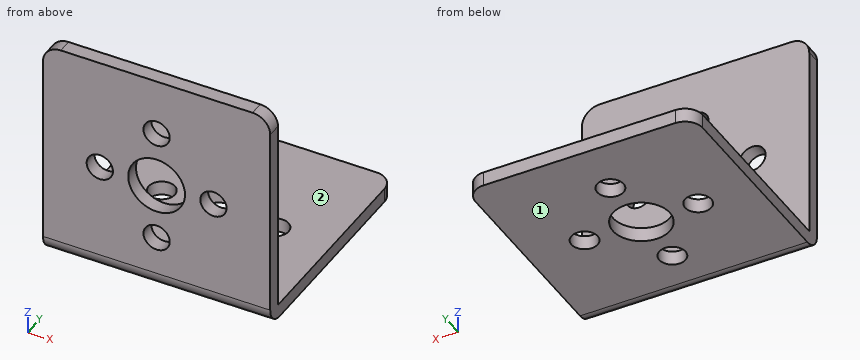
from build123d import *

# Parameters (mm, degrees)
SKETCH1_W           = 32
SKETCH1_H           = 32
BOSS_EXTRUDE1_DEPTH = 16
SKETCH2_W           = 30
SKETCH2_H           = 30
CUT_EXTRUDE1_DEPTH  = 32
SKETCH3_R           = 4
SKETCH3_R_2         = 1.85
CUT_EXTRUDE2_DEPTH  = 33
SKETCH4_R           = 4
SKETCH4_R_2         = 1.85
CUT_EXTRUDE3_DEPTH  = 33
FILLET1_R           = 2.5


with BuildPart() as part:
    # Sketch1 → Boss-Extrude1 (new body, symmetric)
    with BuildSketch(Plane(origin=(0, 0, 0), x_dir=(0, 0, -1), z_dir=(1, 0, 0))):
        Rectangle(SKETCH1_W, SKETCH1_H)
    extrude(amount=BOSS_EXTRUDE1_DEPTH, both=True)

    # Sketch2 → Cut-Extrude1 (cut)
    with BuildSketch(Plane(origin=(16, 0, 0), x_dir=(0, 0, -1), z_dir=(1, 0, 0))):
        with Locations((-1, 1)):
            Rectangle(SKETCH2_W, SKETCH2_H)
    extrude(amount=-CUT_EXTRUDE1_DEPTH, mode=Mode.SUBTRACT)

    # Sketch3 → Cut-Extrude2 (cut, through all)
    with BuildSketch(Plane(origin=(0, 0, -16), x_dir=(-1, 0, 0), z_dir=(0, 0, -1))):
        Circle(SKETCH3_R)
        with Locations((8, 0)):
            Circle(SKETCH3_R_2)
        with Locations((-8, 0)):
            Circle(SKETCH3_R_2)
        with Locations((0, 8)):
            Circle(SKETCH3_R_2)
        with Locations((0, -8)):
            Circle(SKETCH3_R_2)
    extrude(amount=-CUT_EXTRUDE2_DEPTH, mode=Mode.SUBTRACT)

    # Sketch4 → Cut-Extrude3 (cut, through all)
    with BuildSketch(Plane.XZ.offset(16)):
        Circle(SKETCH4_R)
        with Locations((8, 0)):
            Circle(SKETCH4_R_2)
        with Locations((-8, 0)):
            Circle(SKETCH4_R_2)
        with Locations((0, 8)):
            Circle(SKETCH4_R_2)
        with Locations((0, -8)):
            Circle(SKETCH4_R_2)
    extrude(amount=-CUT_EXTRUDE3_DEPTH, mode=Mode.SUBTRACT)

    # Fillet1
    fillet1_edges = [part.edges().sort_by_distance(p)[0] for p in [
        (-16, -15, 16),
        (16, -15, 16),
        (-16, 16, -15),
        (16, 16, -15),
        (0, -16, -16),
    ]]
    fillet(fillet1_edges, radius=FILLET1_R)


solid = part.part
CAD build for the part. Positions are in the model's coordinates, mm. Face numbers are marked on the shaded views. A direction names the side the tool comes from. Round coordinates to 2 decimals unless told otherwise and drop trailing zeros. Write each loop counter-clockwise with the first axis right and the second up, starting at its lowest first coordinate (ties: lowest second). Pieces come first, ordered by that corner, then holes. Notation, with made-up numbers: M 45.25,16.25 L 95.25,16.25 A31 cw 95.25,47.25 Z; hole C 31.5,15 d4. An arc over 180 degrees is marked long. Put each result on its own line as item: value. Start each with the question number.
1) 3-axis set-ups, long thin cutter, end or side, ignore diameter. For the marked faces 1 and 2: which of +Z, -Z, +X, -X, +Y, -Y reach the whole face in a straight line?
2) Pin check, flat tips, straight feed: pin 1 Ø6 at (x, y) = (-8, 0) entering from +Z; pin 2 Ø12 at (x, z) = (-12.5, -4.5) entering from +Y. Stop position of each tip, or through.
3) Saw through at D-D, the plane x = 8. Write the cut outline in (y, z).
4) Drill centre lines: probe 1 along Z at (x, y) = (0, -14.4); probe 2 along Z at (x, y) = (-13, 7.5). Where is each one in solid material? Low to high. Write a range as [from, to].
5) Saw through at A-A, the plane z = 8. Write the cut outline in (x, y).
6) Saw through at B-B, the plane x = 0. Count the separate pieces of the cut face and the enclosed holes in it, and give its area (3 significant figures).
Resolved:
1. face 1: -Z, +X, -X, +Y, -Y
1. face 2: +Z, +X, -X, +Y
2. pin 1: z = -14
2. pin 2: y = -14
3. outline: M -16,-13.5 A2.5 ccw -13.5,-16 L -1.85,-16 L -1.85,-14 L -14,-14 L -14,-1.85 L -16,-1.85 Z; M -16,1.85 L -14,1.85 L -14,16 L -16,16 Z; M 1.85,-16 L 16,-16 L 16,-14 L 1.85,-14 Z
4. probe 1: [-15.83, -9.85], [-6.15, -4], [4, 6.15], [9.85, 16]
4. probe 2: [-16, -14]
5. outline: M -16,-16 L -1.85,-16 L -1.85,-14 L -16,-14 Z; M 1.85,-16 L 16,-16 L 16,-14 L 1.85,-14 Z
6. separate pieces: 7
6. enclosed holes: 0
6. area: 61.1 mm²
